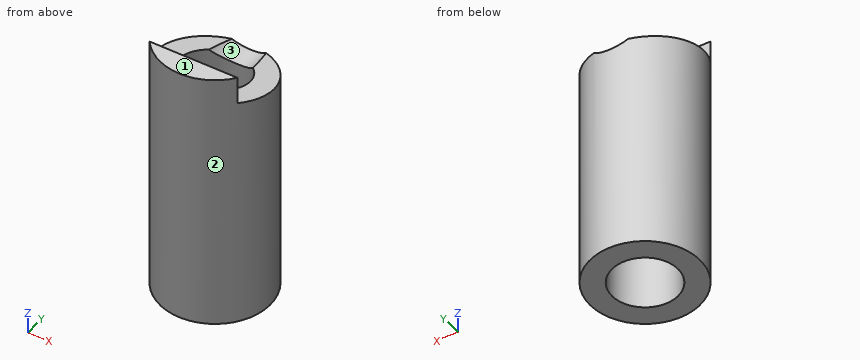
from build123d import *

# Parameters (mm, degrees)
F0_R     = 31.75
F0_R_2   = 19.05
F1_DEPTH = 152.4
F3_DEPTH = 50.8
F4_R     = 15.875
F5_DEPTH = 50.8


with BuildPart() as f1:
    # F0 (on Top) → F1 (new body)
    with BuildSketch(Plane.XY):
        Circle(F0_R)
        Circle(F0_R_2, mode=Mode.SUBTRACT)
    extrude(amount=-F1_DEPTH)

    # F2 (on Right) → F3 (cut, symmetric)
    with BuildSketch(Plane.YZ):
        Polygon((31.75, 0), (-19.05, 0), (-19.05, -15.875), (31.75, -25.4), align=None)
    extrude(amount=F3_DEPTH, both=True, mode=Mode.SUBTRACT)

    # F4 (on Front) → F5 (cut)
    with BuildSketch(Plane.XZ):
        with Locations((0, -12.7)):
            Circle(F4_R)
    extrude(amount=-F5_DEPTH, mode=Mode.SUBTRACT)


solid = f1.part
Could you check a few things on this model? Use its own coordinates, in mm. Face numbers are marked on the shaded views. Round coordinates to 2 decimals unless told otherwise and drop trailing zeros. Loops run counter-clockwise (first coordinate to the right, second up) from the corner with the lowest first, then second, coordinate; pieces in that order, holes last. Notation, with made-up numbers: (73, 77.25) - (102, 77.25) arc R9 cw to (102, 83.25) - close; hole circle Ø3 at (-2.5, 71.5). An arc over 180 degrees is marked (long way). Write item = value, one per line.
1) Imagine slicing it at D-D (y = 16). Please give me the cut outline in (x, z) (3 decimals), and give its area (3 significant figures).
Computed:
outline = (-27.424, -152.4) - (-10.339, -152.4) - (-10.339, -24.746) arc R15.875 cw to (-12.531, -22.447) - (-27.424, -22.447) - close; (10.339, -152.4) - (27.424, -152.4) - (27.424, -22.447) - (12.531, -22.447) arc R15.875 cw to (10.339, -24.746) - close
area = 4,430 mm2
2) I need wall thicknesses on line 1 along Y through (x, z) = (0, -101.5); line 2 along Y through (x, z) = (7, -138). Which ranges of each line are inside material? Lowest first, please. Write a range as from..to.
Computed:
line_1 = -31.75..-19.05, 19.05..31.75
line_2 = -30.97..-17.72, 17.72..30.97
3) I'm going to push flat-ended pins straight in: P1, Ø10, axis at y = -14.5, z = -134, coming from the +X side; P2, Ø6, axis at x = -12.5, z = -78, coming from the -Y side; P3, Ø1, axis at x = -8, z = -97.5, coming from the +Y side; P4, Ø4, axis at x = -13.5, y = -23, coming from the +Z side. Where does each tip first touch, or does it pass through?
Computed:
P1 = 30.3
P2 = -30.3
P3 = 30.85
P4 = 0
4) If we mould it in two halves opening along X, with no side actions, what happens to the marked faces 1, 2 and 3? For each: pulls with the +X half, pulls with the -X half, needs draft (parallel to the pull), parting line crosses it, or undercut.
Computed:
face_1 = needs draft
face_2 = parting line crosses it
face_3 = undercut
5) Imagine slicing it at C-C (z = -84). Please give me the cut outline in (x, y), and give its area (3 significant figures).
Computed:
outline = circle Ø63.5 at (0, 0); hole circle Ø38.1 at (0, 0)
area = 2,030 mm2
6) Imagine slicing it at A-A (x = -2.5). Please give me the cut outline in (y, z) (3 decimals).
Computed:
outline = (-31.651, -152.4) - (-18.885, -152.4) - (-18.885, -15.906) - (-19.05, -15.875) - (-19.05, 0) - (-31.651, 0) - close; (18.885, -152.4) - (31.651, -152.4) - (31.651, -28.377) - (18.885, -28.377) - close
7) Imagine slicing it at B-B (y = -4). Please give me the cut outline in (x, z).
Computed:
outline = (-31.5, -152.4) - (-18.63, -152.4) - (-18.63, -18.7) - (-31.5, -18.7) - close; (18.63, -152.4) - (31.5, -152.4) - (31.5, -18.7) - (18.63, -18.7) - close
